from build123d import *

# Parameters (mm, degrees)
UBODY_SKETCH_R = 5.5
UBODY_DEPTH    = 10.3
TUBE_START     = -13.3
TUBE_SKETCH_R  = 3.175
TUBE_DEPTH     = 13.3
TUBE_RADIUS_R  = 0.5
HEX_2_DEPTH    = 2
HEX_2_DRAFT    = -2
PORT_SKETCH_R  = 2.310158461
PORT_DEPTH     = 18.163624326


with BuildPart() as part:
    # Release_Sketch → Release (revolve)
    with BuildSketch(Plane.XY, mode=Mode.PRIVATE) as release_sk:
        with BuildLine():
            Line((0, 0), (-4.525, 0))
            ThreePointArc((-4.525, 0), (-4.878553391, -0.146446609), (-5.025, -0.5))
            Line((-5.025, -0.5), (-5.025, -1.5))
            Line((-5.025, -1.5), (-3.925, -1.5))
            Line((-3.925, -1.5), (-3.925, -2.4))
            Line((-3.925, -2.4), (0, -2.4))
            Line((0, -2.4), (0, 0))
        make_face()
    revolve(release_sk.sketch.rotate(Axis((0, 0, 0), (0, -1, 0)), 270), axis=Axis((0, 0, 0), (0, -1, 0)))

    # UBody_Sketch → UBody (add)
    with BuildSketch(Plane(origin=(0, -2.4, 0), x_dir=(-1, 0, 0), z_dir=(0, 1, 0))):
        with Locations(Location((0, 0, 0), (0, 0, 90))):
            Circle(UBODY_SKETCH_R)
    extrude(amount=-UBODY_DEPTH)

    # Thread_Sketch → Thread (revolve)
    with BuildSketch(Plane.XY, mode=Mode.PRIVATE) as thread_sk:
        Polygon((-5.247489296, -12.7), (-5.026347442, -19.8), (0, -19.8), (0, -12.7), align=None)
    revolve(thread_sk.sketch.rotate(Axis((0, 0, 0), (0, -1, 0)), 270), axis=Axis((0, 0, 0), (0, -1, 0)))

    # Thread_Chamfer: read off the stored shape, not the designer's step
    # Thread_Chamfer outline → Thread_Chamfer (revolve, cut)
    with BuildSketch(Plane.XY):
        Polygon((5.034384454, -19.541962988), (4.776347442, -19.8), (5.034384454, -19.8), align=None)
    revolve(axis=Axis((0, 0, 0), (0, 1, 0)), mode=Mode.SUBTRACT)

    # Tube_Sketch → Tube (cut)
    with BuildSketch(Plane(origin=(0, 0, 0), x_dir=(1, 0, 0), z_dir=(0, 1, 0)).offset(TUBE_START)):
        with Locations(Location((0, 0, 0), (0, 0, 270))):
            Circle(TUBE_SKETCH_R)
    extrude(amount=TUBE_DEPTH, mode=Mode.SUBTRACT)

    # Tube_Radius
    tube_radius_edges = [part.edges().sort_by_distance(p)[0] for p in [
        (0, 0, -3.175),
    ]]
    fillet(tube_radius_edges, radius=TUBE_RADIUS_R)


with BuildPart() as hex_2_tool:
    # Hex_Sketch → Hex 2 (with draft: the straight prism first)
    with BuildSketch(Plane(origin=(0, -13.3, 0), x_dir=(-1, 0, 0), z_dir=(0, 1, 0))):
        Polygon((-2.748187281, 0), (-1.374093641, -2.38), (1.374093641, -2.38), (2.748187281, 0), (1.374093641, 2.38), (-1.374093641, 2.38), align=None)
    extrude(amount=-HEX_2_DEPTH)
    # Hex 2: the draft: its side faces are tilted about the plane it starts from
    hex_2_sides = [hex_2_tool.faces().sort_by_distance(p)[0] for p in [
        (2.061140461, -14.3, -1.19),
        (0, -14.3, -2.38),
        (-2.061140461, -14.3, -1.19),
        (-2.061140461, -14.3, 1.19),
        (0, -14.3, 2.38),
        (2.061140461, -14.3, 1.19),
    ]]
    draft(hex_2_sides, Plane(origin=(0, -13.3, 0), x_dir=(-1, 0, 0), z_dir=(0, 1, 0)), HEX_2_DRAFT)


with BuildPart() as part_1:
    add(part.part)

    # Hex 2: cut by hex_2_tool
    add(hex_2_tool.part, mode=Mode.SUBTRACT)

    # Port_Sketch → Port (cut, through all)
    with BuildSketch(Plane(origin=(0, -15.3, 0), x_dir=(-1, 0, 0), z_dir=(0, 1, 0))):
        with Locations(Location((0, 0, 0), (0, 0, 90))):
            Circle(PORT_SKETCH_R)
    extrude(amount=-PORT_DEPTH, mode=Mode.SUBTRACT)


solid = part_1.part
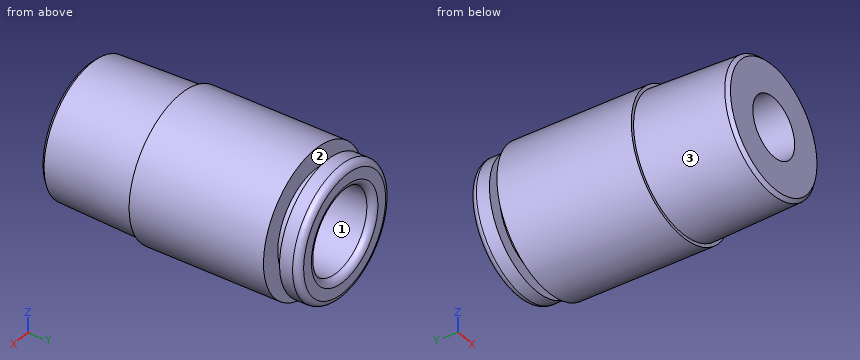
Part model, mm, in its own coordinate system. Face numbers are marked on the shaded views. Give positions to 0.01 mm unless a question says otherwise; leave off trailing zeros. Order: outer loops, then holes, each group sorted by start corner. A loop starts at its lowest first (then second) coordinate and runs counter-clockwise, first axis right, second up. Notation, with made-up numbers: (47, -22) -> (106, -22) arc R21 cw to (106, 0) -> close; hole circle Ø3 at (-2.5, 71.5). An arc over 180 degrees is marked (long way). Use one line per item in the form item = value.
(1) Pull direction Z, two halves, no side cores. Call the marked faces 1, 2 and 3: +Z half, -Z half, draft (parallel to the pull), parting line (faces both ways), or undercut.
Solution:
face_1 = undercut
face_2 = draft
face_3 = parting line
(2) Drill centre lines: line 1 (X direction, y = -5.75, z = 0) (3 decimals); line 2 (Y direction, x = -4.5, z = -0.75); line 3 (Y direction, x = -4.25, z = -3.25). Where is each one in solid material? Low to high. Write a range as from..to.
Solution:
line_1 = -5.5..-3.175, 3.175..5.5
line_2 = -19.8..-2.4, -1.5..0
line_3 = -12.7..-2.4
(3) Saw through at A-A (y = -9.25). Write the cut outline in (x, z) (3 decimals), then the cut area to 3 significant figures.
Solution:
outline = circle Ø11 at (0, 0); hole circle Ø6.35 at (0, 0)
area = 63.4 mm²
(4) Flat gauge pins, fed straight in: P1, Ø3, axis at x = 0, z = 0, coming from the +Y side; P2, Ø0.9, axis at x = -1, z = -2, coming from the +Y side; P3, Ø3, axis at y = -3, z = 2.5, coming from the +X side. Where does each tip first touch, or does it go through?
Solution:
P1 = through
P2 = -13.3
P3 = 5.41
(5) Saw through at B-B (y = -1.75). Write the cut outline in (x, z) (3 decimals).
Solution:
outline = circle Ø7.85 at (0, 0); hole circle Ø6.35 at (0, 0)
